Here's how the part is built. I have some questions about the finished solid (model axes, mm). A direction names the side the tool comes from. Coordinates: 2 decimals unless noted, no trailing zeros. Order: outer loops, then holes, each group sorted by start corner. A loop starts at its lowest first (then second) coordinate and runs counter-clockwise, first axis right, second up. Notation, with made-up numbers: (24, 2.5) -> (59, 2.5) arc R9 ccw to (59, 7.5) -> close; hole circle Ø4 at (-13.5, -0.75). An arc over 180 degrees is marked (long way). One line per item, written item: value. Start each with the question number.
```python
from build123d import *

# Parameters (mm, degrees)
BOSS_EXTRUDE1_DEPTH  = 10
BOSS_EXTRUDE2_START  = 73
BOSS_EXTRUDE2_DEPTH  = 73
SKETCH4_R            = 2.5
BOSS_EXTRUDE3_DEPTH  = 3.9
SKETCH6_R            = 2.45
CUT_EXTRUDE1_DEPTH   = 13.9
SKETCH7_W            = 14
SKETCH7_H            = 20
CUT_EXTRUDE2_DEPTH   = 23.9
BOSS_EXTRUDE4_START  = -3.9
BOSS_EXTRUDE4_DEPTH  = 3.9
SKETCH12_W           = 5
SKETCH12_H           = 10
BOSS_EXTRUDE5_DEPTH  = 0.17
CUT_EXTRUDE3_START   = -73
SKETCH13_R           = 68.75
CUT_EXTRUDE3_DEPTH   = 73
BOSS_EXTRUDE6_DEPTH  = 27
BOSS_EXTRUDE7_DEPTH  = 27
BOSS_EXTRUDE8_DEPTH  = 73
BOSS_EXTRUDE9_START  = -37
BOSS_EXTRUDE9_DEPTH  = 37
BOSS_EXTRUDE10_START = 14
BOSS_EXTRUDE10_DEPTH = 14
CUT_EXTRUDE4_START   = -2
CUT_EXTRUDE4_DEPTH   = 2
SKETCH21_W           = 14
SKETCH21_H           = 20
CUT_EXTRUDE5_DEPTH   = 22
BOSS_EXTRUDE11_START = 14
BOSS_EXTRUDE11_DEPTH = 14
BOSS_EXTRUDE12_START = -5
SKETCH25_R           = 2.45
BOSS_EXTRUDE12_DEPTH = 5
SKETCH24_R           = 2.45
CUT_EXTRUDE6_DEPTH   = 22
BOSS_EXTRUDE13_START = -5
SKETCH26_R           = 2.45
BOSS_EXTRUDE13_DEPTH = 5
BOSS_EXTRUDE14_START = 14
BOSS_EXTRUDE14_DEPTH = 14
SKETCH29_R           = 2.45
CUT_EXTRUDE7_DEPTH   = 22


with BuildPart() as part:
    # Sketch1 → Boss-Extrude1 (new body)
    with BuildSketch(Plane(origin=(0, 0, 0), x_dir=(1, 0, 0), z_dir=(0, 1, 0))):
        with BuildLine():
            Line((0, -67.5), (0, -82.327380707))
            Line((0, -82.327380707), (-5, -82.327380707))
            Line((-5, -82.327380707), (-5, -72.327380707))
            ThreePointArc((-5, -72.327380707), (-72.5, 0), (-5, 72.327380707))
            Line((-5, 72.327380707), (-5, 82.5))
            Line((-5, 82.5), (0, 82.5))
            Line((0, 82.5), (0, 67.5))
            ThreePointArc((0, 67.5), (-67.5, 0), (0, -67.5))
        make_face()
    extrude(amount=BOSS_EXTRUDE1_DEPTH)

    # Sketch2 → Boss-Extrude2 (add)
    with BuildSketch(Plane.XZ.offset(BOSS_EXTRUDE2_START)):
        with BuildLine():
            Line((0, 72.5), (0, 68.5))
            ThreePointArc((0, 68.5), (-68.5, 0), (0, -68.5))
            Line((0, -68.5), (0, -72.5))
            ThreePointArc((0, -72.5), (-72.5, 0), (0, 72.5))
        make_face()
    extrude(amount=-BOSS_EXTRUDE2_DEPTH)

    # Sketch4 → Boss-Extrude3 (add, symmetric)
    # profile 1 of 3: a face of its own
    with BuildSketch(Plane.XZ.offset(73)):
        with BuildLine():
            Line((-70.151512279, 18.30342386), (-87, 18.30342386))
            Line((-87, 18.30342386), (-87, -18.19657614))
            Line((-87, -18.19657614), (-70.179303336, -18.19657614))
            ThreePointArc((-70.179303336, -18.19657614), (-72.499978985, 0.055201399), (-70.151512279, 18.30342386))
        make_face()
        with Locations(Location((-78.75, 10.05342386, 0), (0, 0, 270))):
            Circle(SKETCH4_R, mode=Mode.SUBTRACT)
        with Locations(Location((-78.75, -9.94657614, 0), (0, 0, 270))):
            Circle(SKETCH4_R, mode=Mode.SUBTRACT)
    # profile 2 of 3: a face of its own
    with BuildSketch(Plane.XZ.offset(73)):
        with BuildLine():
            Line((-28.25, -66.769660026), (-28.25, -83.75))
            Line((-28.25, -83.75), (-11.75, -83.75))
            Line((-11.75, -83.75), (-11.75, -71.54150893))
            ThreePointArc((-11.75, -71.54150893), (-20.141813113, -69.645942915), (-28.25, -66.769660026))
        make_face()
        with Locations(Location((-20, -75.5, 0), (0, 0, 270))):
            Circle(SKETCH4_R, mode=Mode.SUBTRACT)
    # profile 3 of 3: a face of its own
    with BuildSketch(Plane.XZ.offset(73)):
        with BuildLine():
            Line((-27, 67.284842275), (-27, 80))
            Line((-27, 80), (-13, 80))
            Line((-13, 80), (-13, 71.324960568))
            ThreePointArc((-13, 71.324960568), (-20.101757111, 69.657514749), (-27, 67.284842275))
        make_face()
        with Locations(Location((-20, 73, 0), (0, 0, 270))):
            Circle(SKETCH4_R, mode=Mode.SUBTRACT)
    extrude(amount=BOSS_EXTRUDE3_DEPTH, both=True)

    # Sketch6 → Cut-Extrude1 (cut)
    with BuildSketch(Plane.ZY.offset(5)):
        with Locations((77.412380707, 5)):
            Circle(SKETCH6_R)
        with Locations((-77.413690354, 5)):
            Circle(SKETCH6_R)
    extrude(amount=-CUT_EXTRUDE1_DEPTH, mode=Mode.SUBTRACT)

    # Sketch7 → Cut-Extrude2 (cut)
    with BuildSketch(Plane.XY.offset(80)):
        with Locations((-20, -59.1)):
            Rectangle(SKETCH7_W, SKETCH7_H)
    extrude(amount=-CUT_EXTRUDE2_DEPTH, mode=Mode.SUBTRACT)

    # Sketch10 → Boss-Extrude4 (add)
    with BuildSketch(Plane(origin=(0, -69.1, 0), x_dir=(1, 0, 0), z_dir=(0, 1, 0)).offset(BOSS_EXTRUDE4_START)):
        with BuildLine():
            Line((-13, -71.324960568), (-13, -75.662480284))
            Line((-13, -75.662480284), (0, -75.662480284))
            Line((0, -75.662480284), (0, -72.5))
            ThreePointArc((0, -72.5), (-6.526498251, -72.205642581), (-13, -71.324960568))
        make_face()
    extrude(amount=BOSS_EXTRUDE4_DEPTH)

    # Sketch12 → Boss-Extrude5 (add)
    with BuildSketch(Plane.XY.offset(82.327380707)):
        with Locations((-2.5, 5)):
            Rectangle(SKETCH12_W, SKETCH12_H)
    extrude(amount=BOSS_EXTRUDE5_DEPTH)

    # Sketch13 → Cut-Extrude3 (cut)
    with BuildSketch(Plane.XZ.offset(73).offset(CUT_EXTRUDE3_START)):
        Circle(SKETCH13_R)
    extrude(amount=CUT_EXTRUDE3_DEPTH, mode=Mode.SUBTRACT)

    # Sketch14 → Boss-Extrude6 (add)
    with BuildSketch(Plane(origin=(0, 10, 0), x_dir=(1, 0, 0), z_dir=(0, 1, 0))):
        with BuildLine():
            Line((-5, -72.327380707), (-5, -82.497380707))
            Line((-5, -82.497380707), (0, -82.497380707))
            Line((0, -82.497380707), (0, -67.5))
            ThreePointArc((0, -67.5), (-67.5, 0), (0, 67.5))
            Line((0, 67.5), (0, 82.5))
            Line((0, 82.5), (-5, 82.5))
            Line((-5, 82.5), (-5, 72.327380707))
            ThreePointArc((-5, 72.327380707), (-72.5, 0), (-5, -72.327380707))
        make_face()
    extrude(amount=BOSS_EXTRUDE6_DEPTH)

    # Sketch15 → Boss-Extrude7 (add)
    with BuildSketch(Plane(origin=(0, 37, 0), x_dir=(1, 0, 0), z_dir=(0, 1, 0))):
        with BuildLine():
            Line((0, 68.2), (0, 72.5))
            ThreePointArc((0, 72.5), (-72.5, 0), (0, -72.5))
            Line((0, -72.5), (0, -68.2))
            ThreePointArc((0, -68.2), (-68.2, 0), (0, 68.2))
        make_face()
    extrude(amount=BOSS_EXTRUDE7_DEPTH)

    # Sketch17 → Boss-Extrude8 (add)
    with BuildSketch(Plane.XZ):
        with BuildLine():
            Line((0, 68.2), (0, 68.75))
            ThreePointArc((0, 68.75), (-68.75, 0), (0, -68.75))
            Line((0, -68.75), (0, -68.2))
            ThreePointArc((0, -68.2), (-68.2, 0), (0, 68.2))
        make_face()
    extrude(amount=BOSS_EXTRUDE8_DEPTH)

    # Sketch18 → Boss-Extrude9 (add)
    with BuildSketch(Plane(origin=(0, 37, 0), x_dir=(1, 0, 0), z_dir=(0, 1, 0)).offset(BOSS_EXTRUDE9_START)):
        with BuildLine():
            Line((0, -67.25), (0, -67.5))
            ThreePointArc((0, -67.5), (-67.5, 0), (0, 67.5))
            Line((0, 67.5), (0, 67.25))
            ThreePointArc((0, 67.25), (-67.25, 0), (0, -67.25))
        make_face()
    extrude(amount=BOSS_EXTRUDE9_DEPTH)

    # Sketch19 → Boss-Extrude10 (add)
    with BuildSketch(Plane.XZ.offset(BOSS_EXTRUDE10_START)):
        with BuildLine():
            Line((0, -68.2), (0, -67.25))
            ThreePointArc((0, -67.25), (-67.25, 0), (0, 67.25))
            Line((0, 67.25), (0, 68.2))
            ThreePointArc((0, 68.2), (-68.2, 0), (0, -68.2))
        make_face()
    extrude(amount=-BOSS_EXTRUDE10_DEPTH)

    # Sketch20 → Cut-Extrude4 (cut)
    with BuildSketch(Plane(origin=(0, 37, 0), x_dir=(1, 0, 0), z_dir=(0, 1, 0)).offset(CUT_EXTRUDE4_START)):
        with BuildLine():
            Line((0, 67.25), (0, 68.2))
            ThreePointArc((0, 68.2), (-68.2, 0), (0, -68.2))
            Line((0, -68.2), (0, -67.25))
            ThreePointArc((0, -67.25), (-67.25, 0), (0, 67.25))
        make_face()
    extrude(amount=CUT_EXTRUDE4_DEPTH, mode=Mode.SUBTRACT)

    # Sketch21 → Cut-Extrude5 (cut)
    with BuildSketch(Plane.XY.offset(80)):
        with Locations((-20, -59.1)):
            Rectangle(SKETCH21_W, SKETCH21_H)
    extrude(amount=-CUT_EXTRUDE5_DEPTH, mode=Mode.SUBTRACT)

    # Sketch23 → Boss-Extrude11 (add)
    with BuildSketch(Plane.XZ.offset(BOSS_EXTRUDE11_START)):
        with BuildLine():
            Line((0, 72.5), (0, 82.497380707))
            Line((0, 82.497380707), (-5, 82.497380707))
            Line((-5, 82.497380707), (-5, 72.327380707))
            ThreePointArc((-5, 72.327380707), (-2.501489427, 72.456832325), (0, 72.5))
        make_face()
    extrude(amount=-BOSS_EXTRUDE11_DEPTH)

    # Sketch25 → Boss-Extrude12 (add)
    with BuildSketch(Plane(origin=(0, 0, 0), x_dir=(0, 0, -1), z_dir=(1, 0, 0)).offset(BOSS_EXTRUDE12_START)):
        with Locations((-77.412380707, 5)):
            Circle(SKETCH25_R)
    extrude(amount=BOSS_EXTRUDE12_DEPTH)

    # Sketch24 → Cut-Extrude6 (cut)
    with BuildSketch(Plane(origin=(0, 0, 0), x_dir=(0, 0, -1), z_dir=(1, 0, 0))):
        with Locations((-77.412380707, -9.05)):
            Circle(SKETCH24_R)
        with Locations((-77.412380707, 32.05)):
            Circle(SKETCH24_R)
        with Locations((-77.412380707, 11.5)):
            Circle(SKETCH24_R)
    extrude(amount=-CUT_EXTRUDE6_DEPTH, mode=Mode.SUBTRACT)

    # Sketch26 → Boss-Extrude13 (add)
    with BuildSketch(Plane(origin=(0, 0, 0), x_dir=(0, 0, -1), z_dir=(1, 0, 0)).offset(BOSS_EXTRUDE13_START)):
        with Locations((77.413690354, 5)):
            Circle(SKETCH26_R)
    extrude(amount=BOSS_EXTRUDE13_DEPTH)

    # Sketch27 → Boss-Extrude14 (add)
    with BuildSketch(Plane.XZ.offset(BOSS_EXTRUDE14_START)):
        with BuildLine():
            Line((-5, -72.327380707), (-5, -82.5))
            Line((-5, -82.5), (0, -82.5))
            Line((0, -82.5), (0, -72.5))
            ThreePointArc((0, -72.5), (-2.501489427, -72.456832325), (-5, -72.327380707))
        make_face()
    extrude(amount=-BOSS_EXTRUDE14_DEPTH)

    # Sketch29 → Cut-Extrude7 (cut)
    with BuildSketch(Plane(origin=(0, 0, 0), x_dir=(0, 0, -1), z_dir=(1, 0, 0))):
        with Locations((77.41, 32.05)):
            Circle(SKETCH29_R)
        with Locations((77.41, 11.5)):
            Circle(SKETCH29_R)
        with Locations((77.41, -9.05)):
            Circle(SKETCH29_R)
    extrude(amount=-CUT_EXTRUDE7_DEPTH, mode=Mode.SUBTRACT)


solid = part.part
```
Q1. Imagine slicing it at B-B (y = 11.5). Write out the boundary of the cut face in (x, z).
Q2. Imagine slicing it at A-A (y = -57). Write out the boundary of the cut face in (x, z), plus the area to 3 significant figures.
Q3. For P1, Ø1, axis at x = -44.5, y = -32, coming from the -Z side; P2, Ø5, axis at y = -56, z = 69, coming from the -X side; P3, Ø6, axis at x = -80, y = -72, coming from the +Z side, each with a flat end and sliding along its axis, tell me the tip position at first contact or that it passes through.
Q4. Imagine slicing it at D-D (z = -56). Write out the boundary of the cut face in (x, y).
Q5. I need wall thicknesses on line 1 (Y direction, x = -4, z = -77); line 2 (Y direction, x = -72, z = -15.5); line 3 (Z direction, x = -7.5, y = -17). Which ranges of each line are inside material? Lowest first, please.
Q6. For faces 4 (the face through (-79, -73, -18.197)), 5 (the face through (-69, -73, 2)), 6 (the face through (-78, -73, 18.303)), 7 (the face through (-2.465, 11.608, -74.962)), 8 (the face through (-67, 35, -10)), which set-ups out of +Z, -Z, +X, -X, +Y, -Y let a thin tool reach every point of the face, with its end or its side?
Q7. If we mould it in two halves opening along X, with no side actions, what happens to faces 1 (the face through (-87, -73, 0)), 2 (the face through (-67.234, 10.157, -1.479)), 3 (the face through (-20, -73, -73))? For each: +X half, -X half, draft (parallel to the pull), parting line (faces both ways), or undercut.
Q8. Imagine slicing it at C-C (x = -20). Count the separate pieces of the cut face and the enclosed holes in it, plus the area to 3 significant figures.
Completed:
1. outline: (-5, -82.5) -> (0, -82.5) -> (0, -79.86) -> (-5, -79.86) -> close; (-5, -74.96) -> (0, -74.96) -> (0, -67.25) arc R67.25 cw to (0, 67.25) -> (0, 74.96) -> (-5, 74.96) -> (-5, 72.33) arc R72.5 ccw to (-5, -72.33) -> close; (-5, 79.86) -> (0, 79.86) -> (0, 82.5) -> (-5, 82.5) -> close
2. outline: (-27, 62.63) -> (-27, 67.28) arc R72.5 ccw to (0, -72.5) -> (0, -68.2) arc R68.2 cw to start; (-13, 66.95) arc R68.2 cw to (0, 68.2) -> (0, 72.5) arc R72.5 ccw to (-13, 71.32) -> close
2. area: 887 mm2
3. P1: stops at z = -57.62
3. P2: stops at x = -28.88
3. P3: stops at z = 18.3
4. outline: (-46.05, -73) -> (-38.93, -73) -> (-38.93, -14) -> (-37.24, -14) -> (-37.24, 35) -> (-38.93, 35) -> (-38.93, 64) -> (-46.05, 64) -> close
5. line 1: y = -14 to -11.47, -6.63 to 9.08, 13.92 to 29.63, 34.47 to 37
5. line 2: y = -76.9 to -69.1
5. line 3: z = -72.11 to -67.79, 67.79 to 72.11
6. face 4: -Z, -X, +Y, -Y
6. face 5: +X, -Y
6. face 6: +Z, -X, +Y, -Y
6. face 7: +X, -X
6. face 8: +X, +Y
7. face 1: -X half
7. face 2: +X half
7. face 3: undercut
8. separate pieces: 5
8. enclosed holes: 0
8. area: 1,350 mm2
